```python
from build123d import *

# Parameters (mm, degrees)
ESQUISSE1_R        = 6
ESQUISSE1_R_2      = 5
BOSS_EXTRU_1_DEPTH = 10
ESQUISSE2_R        = 6
ESQUISSE2_R_2      = 4.5
BOSS_EXTRU_2_DEPTH = 1
ESQUISSE3_R        = 9
ESQUISSE3_R_2      = 5
BOSS_EXTRU_3_DEPTH = 2
ESQUISSE4_R        = 5.5
ESQUISSE4_R_2      = 5
BOSS_EXTRU_4_DEPTH = 2
ESQUISSE5_R        = 6
ESQUISSE5_R_2      = 5
BOSS_EXTRU_5_DEPTH = 10
ESQUISSE6_R        = 6
ESQUISSE6_R_2      = 5
BOSS_EXTRU_6_DEPTH = 10


with BuildPart() as part:
    # Esquisse1 → Boss.-Extru.1 (new body)
    with BuildSketch(Plane.XY):
        Circle(ESQUISSE1_R)
        Circle(ESQUISSE1_R_2, mode=Mode.SUBTRACT)
    extrude(amount=BOSS_EXTRU_1_DEPTH)

    # Esquisse2 → Boss.-Extru.2 (add)
    with BuildSketch(Plane(origin=(0, 0, 0), x_dir=(-1, 0, 0), z_dir=(0, 0, -1))):
        Circle(ESQUISSE2_R)
        Circle(ESQUISSE2_R_2, mode=Mode.SUBTRACT)
    extrude(amount=BOSS_EXTRU_2_DEPTH)

    # Esquisse3 → Boss.-Extru.3 (add)
    with BuildSketch(Plane.XY.offset(10)):
        Circle(ESQUISSE3_R)
        Circle(ESQUISSE3_R_2, mode=Mode.SUBTRACT)
    extrude(amount=BOSS_EXTRU_3_DEPTH)

    # Esquisse4 → Boss.-Extru.4 (add)
    with BuildSketch(Plane.XY.offset(12)):
        Circle(ESQUISSE4_R)
        Circle(ESQUISSE4_R_2, mode=Mode.SUBTRACT)
    extrude(amount=BOSS_EXTRU_4_DEPTH)

    # Esquisse5 → Boss.-Extru.5 (add)
    with BuildSketch(Plane.XY.offset(14)):
        Circle(ESQUISSE5_R)
        Circle(ESQUISSE5_R_2, mode=Mode.SUBTRACT)
    extrude(amount=BOSS_EXTRU_5_DEPTH)

    # Esquisse6 → Boss.-Extru.6 (add)
    with BuildSketch(Plane.XY.offset(24)):
        Circle(ESQUISSE6_R)
        Circle(ESQUISSE6_R_2, mode=Mode.SUBTRACT)
    extrude(amount=BOSS_EXTRU_6_DEPTH)


solid = part.part
```
Input: part model. Units: mm. Frame: model coordinates. A direction names the side the tool comes from. Coordinates: 2 decimals unless noted, no trailing zeros. Loops run counter-clockwise (first coordinate to the right, second up) from the corner with the lowest first, then second, coordinate; pieces in that order, holes last. Notation, with made-up numbers: M -29.5,-21.75 L -21.5,-21.75 A14 ccw -21.5,1.25 Z; hole C -4.5,-31 d7. An arc over 180 degrees is marked long. Answer in a Markdown table with one row per item.
1. Reachability of faces 4 (the cylindrical face through (-1.19, -5.37, 12.99)), 5 (the flat face through (2, -6, 10)), 6 (the flat face through (1.4, 4.5, -1)) from +Z, -Z, +X, -X, +Y, -Y: full face, straight path, thin tool, end or side. Return the list, or none.
Response:
| item | result |
|---|---|
| face 4 | none |
| face 5 | -Z |
| face 6 | -Z, +X, -X, +Y, -Y |
2. First-contact query: pin 1 (8 mm diameter, centred on y = -3, z = 24.5, fed in from +X); pin 2 (10 mm diameter, centred on x = -7, z = 11, fed in from +Y); pin 3 (4 mm diameter, centred on y = 1, z = 24, fed in from -X). Flat tips, straight axial feed; report the tip coordinate or a pass-through.
Response:
| item | result |
|---|---|
| pin 1 | stops at x = 6 |
| pin 2 | stops at y = 8.77 |
| pin 3 | stops at x = -6 |
3. Section C-C, the plane z = 3. Output: boundary loops of the cut face in (x, y).
Response:
| item | result |
|---|---|
| outline | C 0,0 d12; hole C 0,0 d10 |
4. Draft query along Y for faces 1 (the cylindrical face through (-6, 0, 24)), 2 (the cylindrical face through (-1.08, -4.88, 16.76)), 3 (the flat face through (3, -5, 14)). Return one class per face: pulls with the +Y half, pulls with the -Y half, needs draft (parallel to the pull), parting line crosses it, or undercut.
Response:
| item | result |
|---|---|
| face 1 | parting line crosses it |
| face 2 | undercut |
| face 3 | needs draft |
5. Section A-A, the plane y = 0. Output: boundary loops of the cut face in (x, z), then the cut area to 3 significant figures.
Response:
| item | result |
|---|---|
| outline | M -9,10 L -6,10 L -6,-1 L -4.5,-1 L -4.5,0 L -5,0 L -5,34 L -6,34 L -6,14 L -5.5,14 L -5.5,12 L -9,12 Z; M 4.5,-1 L 6,-1 L 6,10 L 9,10 L 9,12 L 5.5,12 L 5.5,14 L 6,14 L 6,34 L 5,34 L 5,0 L 4.5,0 Z |
| area | 81.0 mm2 |
6. Section D-D, the plane z = 12.5. Output: boundary loops of the cut face in (x, y).
Response:
| item | result |
|---|---|
| outline | C 0,0 d11; hole C 0,0 d10 |
7. Material intervals for line 1 (Y direction, x = -0.25, z = 21); line 2 (Y direction, x = 0, z = -0.7); line 3 (Z direction, x = 4, y = -5.5), sorted ascending.
Response:
| item | result |
|---|---|
| line 1 | y = -5.99 to -4.99, 4.99 to 5.99 |
| line 2 | y = -6 to -4.5, 4.5 to 6 |
| line 3 | z = 10 to 12 |
